Geometry check sheet. Reference: the model listing, model coordinates, mm. Face numbers are marked on the shaded views. A direction names the side the tool comes from. Round coordinates to 2 decimals unless told otherwise and drop trailing zeros. Order: outer loops, then holes, each group sorted by start corner. A loop starts at its lowest first (then second) coordinate and runs counter-clockwise, first axis right, second up.
(1) Cross-section at B-B on z = 0. Enter the section's corners in (x, y).
(2) Gauge pin test, flat ends, axial feed: P1, Ø1, axis at x = 4, z = 3.5, coming from the +Y side; P2, Ø8, axis at y = 21.5, z = -1.5, coming from the -X side; P3, Ø1, axis at y = 59, z = -0.5, coming from the +X side; P4, Ø2, axis at x = -1, y = 31, coming from the -Z side. Record the tip position at first contact, or that the pin passes through.
(3) Set-up check for the marked faces 1, 2 and 3: record each of +Z, -Z, +X, -X, +Y, -Y from which the full face is reachable in a straight line by a thin tool's end or side.
(4) Thickness scan on L1, parallel to Y at x = -0.25, z = 4.75; L2, parallel to Y at x = -3, z = 6; L3, parallel to Y at x = -3.5, z = -7.5. Record the ranges inside material, lowest first.
(5) Cross-section at A-A on y = 16. Enter the section's corners in (x, z).
(6) Cross-section at C-C on y = 31. Enter the section's corners in (x, z), and give its area (3 significant figures).
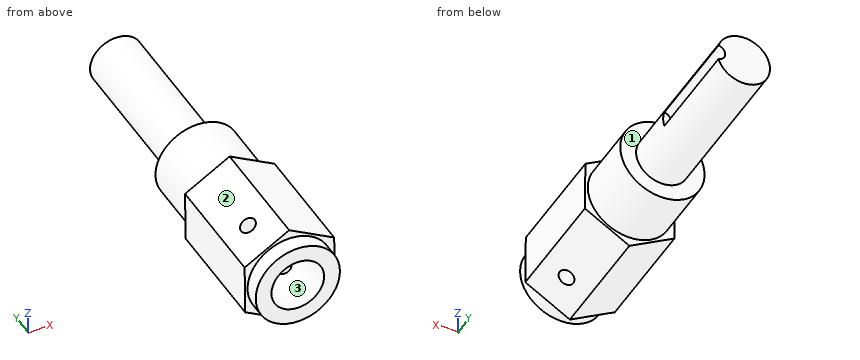
Autodesk Inventor part; units mm, degrees
ref_plane "YZ Plane" through (0, 0, 0) normal (1, 0, 0) x (0, 1, 0)
ref_plane "XZ Plane" through (0, 0, 0) normal (0, 1, 0) x (-1, 0, 0)
ref_plane "XY Plane" through (0, 0, 0) normal (0, 0, 1) x (1, 0, 0)
sketch "Sketch1" plane through (0, 0, 0) normal (0, 1, 0) x (-1, 0, 0)
  line L0 (8.5475, 4.8243) -> (8.4517, -4.9902)
  line L1 (8.4517, -4.9902) -> (-0.0957, -9.8145)
  line L2 (-0.0957, -9.8145) -> (-8.5475, -4.8243)
  line L3 (-8.5475, -4.8243) -> (-8.4517, 4.9902)
  line L4 (-8.4517, 4.9902) -> (0.0957, 9.8145)
  line L5 (0.0957, 9.8145) -> (8.5475, 4.8243)
  circle A0 centre (0, 0) radius 5
  dimension "d0" = 17
  dimension "d1" = 10
extrude "Extrusion1" add sketch "Sketch1" along normal blind 37
sketch "Sketch2" plane through (0, 37, 0) normal (0, 1, 0) x (1, 0, 0)
  circle A0 centre (0, 0) radius 8
  circle A1 centre (0, 0) radius 13
  circle A2 centre (0, 0) radius 5
  dimension "d4" = 16
  dimension "d5" = 5
extrude "Extrusion2" cut sketch "Sketch2" against normal blind 12 contours A1
sketch "Sketch3" plane through (0, 0, 0) normal (0, -1, 0) x (1, 0, 0)
  circle A0 centre (0, 0) radius 8
  circle A1 centre (0, 0) radius 13
  dimension "d9" = 16
  dimension "d10" = 5
extrude "Extrusion3" cut sketch "Sketch3" against normal blind 3
sketch "Sketch9" plane through (0.0957, 3, -9.8145) normal (0.5084, 0, -0.8611) x (-0.8611, 0, -0.5084)
  circle A0 centre (-4.9075, 7) radius 1.5
  line L0 (-9.815, 0) -> (-9.815, 22)
  line L1 (0, 0) -> (0, 22)
  point P0 (-4.9075, -3)
  dimension "d31" = 3
  dimension "d32" = 9.8149
  dimension "d33" = 4.9075
  dimension "d34" = 10
extrude "Extrusion5" cut sketch "Sketch9" against normal through all
extrude "Extrusion6" add sketch "Sketch2" along normal blind 30 and the other way blind 5 contours A2
sketch "Sketch10" plane through (0, 67, 0) normal (0, 1, 0) x (1, 0, 0)
  circle A0 centre (0, 0) radius 5
  circle A1 centre (5, 0) radius 1.5
  dimension "d45" = 3
extrude "Extrusion7" cut sketch "Sketch10" against normal blind 20 contours A0 A1 | A0 A1 picked at (4.5056, -0.2843) picked at (5.4323, -0.4031)
equation "\"d33\" = 0.5 * d32"
properties part number "AnyaKicsi"
Found:
1. outline: (-8.5, 3) - (-8, 3) - (-8, 0) - (-5, 0) - (-5, 32) - (5, 32) - (5, 0) - (8, 0) - (8, 3) - (8.5, 3) - (8.5, 25) - (8, 25) - (8, 37) - (5, 37) - (5, 47) - (3.5, 47) - (3.5, 67) - (-5, 67) - (-5, 37) - (-8, 37) - (-8, 25) - (-8.5, 25) - close
2. P1: stops at y = 67
2. P2: stops at x = -8.52
2. P3: stops at x = 3.88
2. P4: stops at z = -8
3. face 1: +Y
3. face 2: +Z, -X, +Y, -Y
3. face 3: -Y
4. L1: y = 32 to 67
4. L2: y = 0 to 8.57, 11.43 to 37
4. L3: y = 3 to 25
5. outline: (-8.55, 4.82) - (-8.45, -4.99) - (0.1, -9.81) - (8.55, -4.82) - (8.45, 4.99) - (-0.1, 9.81) - close; hole circle Ø10 at (0, 0)
6. outline: circle Ø16 at (0, 0); hole circle Ø10 at (0, 0)
6. area: 123 mm2
